Can you work these out from the drawing? Everything is in mm from the part's minimum corner. A direction names the side the tool comes from. Round coordinates to 2 decimals unless told otherwise and drop trailing zeros. Write each loop counter-clockwise with the first axis right and the second up, starting at its lowest first coordinate (ties: lowest second). Pieces come first, ordered by that corner, then holes. Notation, with made-up numbers: (34.5, 62) - (73.5, 62) arc R28 cw to (73.5, 85) - close; hole circle Ø1 at (17.5, 10.5). An arc over 180 degrees is marked (long way). One line per item, written item: value. Start each with the question number.
(1) I want a section at A-A on z = 15.25. List the corners of the cut face in (x, y) for me.
(2) On a 3-axis mill with a long thin cutter (end or side, diameter ignored), from which of +Z, -Z, +X, -X, +Y, -Y can I reach the whole of each face in a straight line? I mean the marked faces 5 and 6. Say none if no direction works.
(3) I want a section at C-C on y = 4.25. List the corners of the cut face in (x, z) for me.
(4) I want a section at D-D on x = 11. List the corners of the cut face in (y, z) for me.
(5) Thinking about a two-plate mould opening in Y: for the marked faces 1, 2, 3 and 4, which applies, +Y half, -Y half, draft (parallel to the pull), parting line (faces both ways), or undercut?
(6) I want a section at B-B on x = 2.5. List the corners of the cut face in (y, z) for me.
(7) I'm going to push flat-ended pins straight in: pin 1 Ø0.6 at (x, y) = (7, 1) entering from -Z; pin 2 Ø3 at (y, z) = (6, 7.5) entering from +X. Where does each tip first touch, or does it pass through?
(8) If I drill on L1, parallel to Z at x = 14, y = 4; L2, parallel to X at y = 1, z = 5; L3, parallel to Y at x = 14.5, z = 10.25, over which ranges is the centre line in solid material (lowest first)? Write a range as from..to.
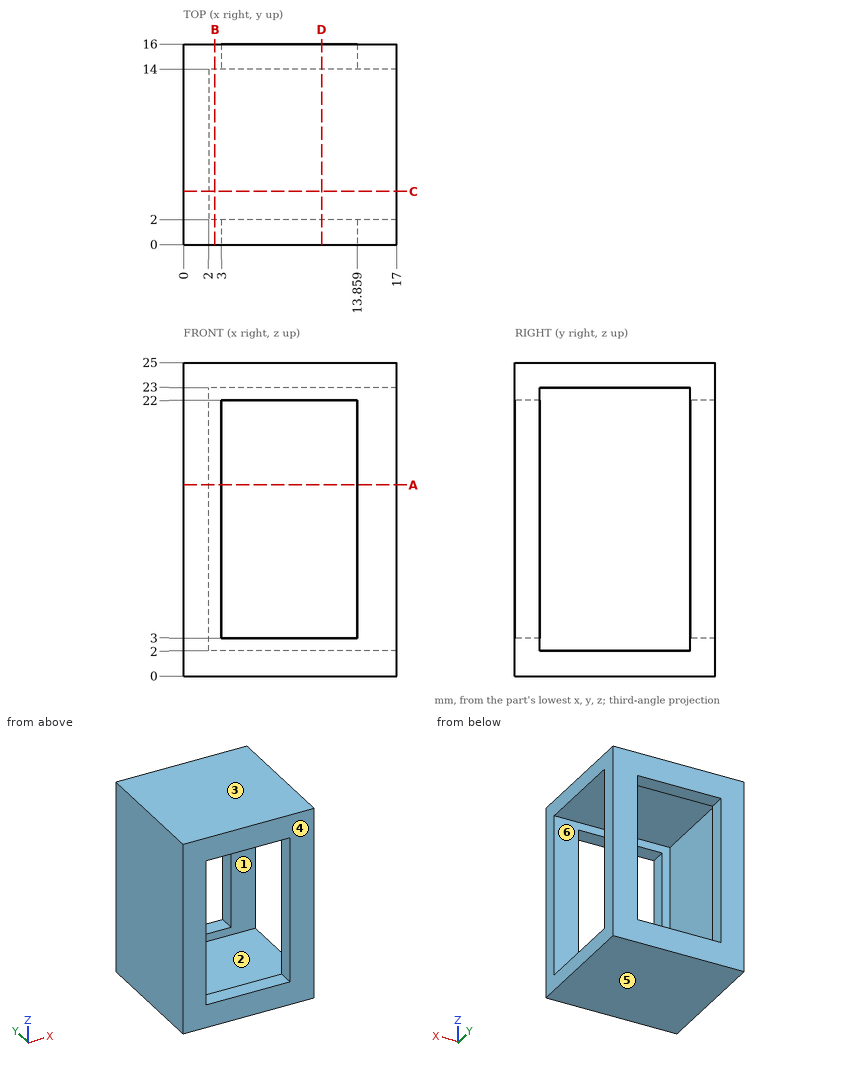
Established:
1. outline: (0, 0) - (3, 0) - (3, 2) - (2, 2) - (2, 14) - (3, 14) - (3, 16) - (0, 16) - close; (13.86, 0) - (17, 0) - (17, 2) - (13.86, 2) - close; (13.86, 14) - (17, 14) - (17, 16) - (13.86, 16) - close
2. face 5: -Z, +X, -X, +Y, -Y
2. face 6: +X
3. outline: (0, 0) - (17, 0) - (17, 2) - (2, 2) - (2, 23) - (17, 23) - (17, 25) - (0, 25) - close
4. outline: (0, 0) - (16, 0) - (16, 3) - (14, 3) - (14, 2) - (2, 2) - (2, 3) - (0, 3) - close; (0, 22) - (2, 22) - (2, 23) - (14, 23) - (14, 22) - (16, 22) - (16, 25) - (0, 25) - close
5. face 1: undercut
5. face 2: undercut
5. face 3: draft
5. face 4: -Y half
6. outline: (0, 0) - (16, 0) - (16, 25) - (0, 25) - close; hole (2, 2) - (14, 2) - (14, 23) - (2, 23) - close
7. pin 1: z = 0
7. pin 2: x = 2
8. L1: 0..2, 23..25
8. L2: 0..3, 13.86..17
8. L3: 0..2, 14..16
